```python
from build123d import *

# Parameters (mm, degrees)
F0_R     = 609.6
F0_R_2   = 4.826
F0_R_3   = 3.175
F0_R_4   = 44.9961
F1_DEPTH = 6.35


with BuildPart() as f1:
    # F0 (on Top) → F1 (new body)
    with BuildSketch(Plane.XY):
        Circle(F0_R)
        with Locations((-383.730187, -440.500605)):
            Circle(F0_R_2, mode=Mode.SUBTRACT)
        with Locations((-441.988335, -382.015644)):
            Circle(F0_R_2, mode=Mode.SUBTRACT)
        with Locations((-42.407097, -582.658801)):
            Circle(F0_R_2, mode=Mode.SUBTRACT)
        with Locations((-582.819183, -40.142748)):
            Circle(F0_R_2, mode=Mode.SUBTRACT)
        with Locations((-1.195725, -177.795979)):
            Circle(F0_R_2, mode=Mode.SUBTRACT)
        with Locations((-126.566248, -124.875237)):
            Circle(F0_R_2, mode=Mode.SUBTRACT)
        with Locations((-76.57454, -133.362918)):
            Circle(F0_R_2, mode=Mode.SUBTRACT)
        with Locations((-136.75852, -76.588043)):
            Circle(F0_R_2, mode=Mode.SUBTRACT)
        with Locations((-42.546952, -150.858801)):
            Circle(F0_R_2, mode=Mode.SUBTRACT)
        with Locations((-148.4482, -40.155448)):
            Circle(F0_R_2, mode=Mode.SUBTRACT)
        with Locations((-47.623603, -27.4955)):
            Circle(F0_R_3, mode=Mode.SUBTRACT)
        with Locations((40.142748, -582.819183)):
            Circle(F0_R_2, mode=Mode.SUBTRACT)
        with Locations((382.015644, -441.988335)):
            Circle(F0_R_2, mode=Mode.SUBTRACT)
        with Locations((440.500605, -383.730187)):
            Circle(F0_R_2, mode=Mode.SUBTRACT)
        with Locations((40.155448, -148.4482)):
            Circle(F0_R_2, mode=Mode.SUBTRACT)
        with Locations((76.588043, -136.75852)):
            Circle(F0_R_2, mode=Mode.SUBTRACT)
        with Locations((124.875237, -126.566248)):
            Circle(F0_R_2, mode=Mode.SUBTRACT)
        with Locations((133.362918, -76.57454)):
            Circle(F0_R_2, mode=Mode.SUBTRACT)
        with Locations((0, -54.991)):
            Circle(F0_R_3, mode=Mode.SUBTRACT)
        with Locations((47.623603, -27.4955)):
            Circle(F0_R_3, mode=Mode.SUBTRACT)
        with Locations((150.858801, -42.546952)):
            Circle(F0_R_2, mode=Mode.SUBTRACT)
        with Locations((177.795979, -1.195725)):
            Circle(F0_R_2, mode=Mode.SUBTRACT)
        with Locations((582.658801, -42.407097)):
            Circle(F0_R_2, mode=Mode.SUBTRACT)
        with Locations((-582.658801, 42.407097)):
            Circle(F0_R_2, mode=Mode.SUBTRACT)
        with Locations((-177.795979, 1.195725)):
            Circle(F0_R_2, mode=Mode.SUBTRACT)
        with Locations((-150.858801, 42.546952)):
            Circle(F0_R_2, mode=Mode.SUBTRACT)
        with Locations((-47.623603, 27.4955)):
            Circle(F0_R_3, mode=Mode.SUBTRACT)
        with Locations((-133.362918, 76.57454)):
            Circle(F0_R_2, mode=Mode.SUBTRACT)
        with Locations((-124.875237, 126.566248)):
            Circle(F0_R_2, mode=Mode.SUBTRACT)
        with Locations((-76.588043, 136.75852)):
            Circle(F0_R_2, mode=Mode.SUBTRACT)
        with Locations((-40.155448, 148.4482)):
            Circle(F0_R_2, mode=Mode.SUBTRACT)
        with Locations((-440.500605, 383.730187)):
            Circle(F0_R_2, mode=Mode.SUBTRACT)
        with Locations((-382.015644, 441.988335)):
            Circle(F0_R_2, mode=Mode.SUBTRACT)
        with Locations((-40.142748, 582.819183)):
            Circle(F0_R_2, mode=Mode.SUBTRACT)
        Circle(F0_R_4, mode=Mode.SUBTRACT)
        with Locations((47.623603, 27.4955)):
            Circle(F0_R_3, mode=Mode.SUBTRACT)
        with Locations((0, 54.991)):
            Circle(F0_R_3, mode=Mode.SUBTRACT)
        with Locations((148.4482, 40.155448)):
            Circle(F0_R_2, mode=Mode.SUBTRACT)
        with Locations((42.546952, 150.858801)):
            Circle(F0_R_2, mode=Mode.SUBTRACT)
        with Locations((136.75852, 76.588043)):
            Circle(F0_R_2, mode=Mode.SUBTRACT)
        with Locations((76.57454, 133.362918)):
            Circle(F0_R_2, mode=Mode.SUBTRACT)
        with Locations((126.566248, 124.875237)):
            Circle(F0_R_2, mode=Mode.SUBTRACT)
        with Locations((1.195725, 177.795979)):
            Circle(F0_R_2, mode=Mode.SUBTRACT)
        with Locations((582.819183, 40.142748)):
            Circle(F0_R_2, mode=Mode.SUBTRACT)
        with Locations((42.407097, 582.658801)):
            Circle(F0_R_2, mode=Mode.SUBTRACT)
        with Locations((441.988335, 382.015644)):
            Circle(F0_R_2, mode=Mode.SUBTRACT)
        with Locations((383.730187, 440.500605)):
            Circle(F0_R_2, mode=Mode.SUBTRACT)
    extrude(amount=F1_DEPTH)


solid = f1.part
```
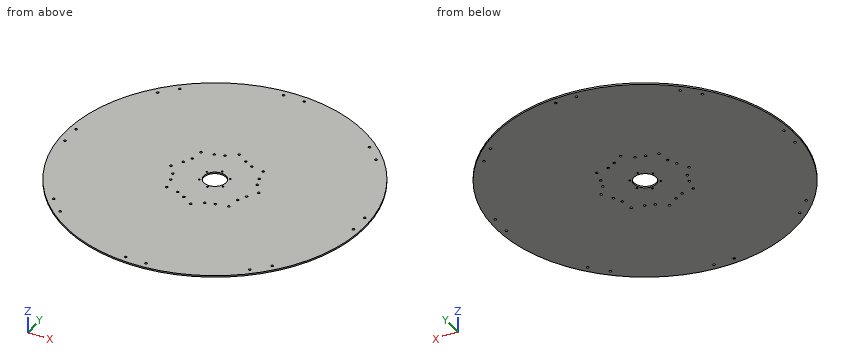
Work out the finished part from the listing and answer in its coordinate system (mm). Round coordinates to 2 decimals unless told otherwise and drop trailing zeros. Loops run counter-clockwise (first coordinate to the right, second up) from the corner with the lowest first, then second, coordinate; pieces in that order, holes last. Notation, with made-up numbers: M -12.75,61 L 34.25,61 A11 ccw 34.25,82 Z; hole C -28,-24.75 d7. An arc over 180 degrees is marked long. One line per question, with ' | ' between items.
Q1. Find section B-B, the plane y = 226. Give the vertices of the cut face in (x, z).
Conclusion:
outline: M -566.16,0 L 566.16,0 L 566.16,6.35 L -566.16,6.35 Z
Q2. Find section C-C, the plane z = 4. State how many separate pieces and enclosed holes the cut face has, then the cut area to 3 significant figures.
Conclusion:
separate pieces: 1 | enclosed holes: 47 | area: 1,160,000 mm2
Q3. Find section A-A, the plane x = -523.5. Give the vertices of the cut face in (y, z), then the cut area to 3 significant figures.
Conclusion:
outline: M -312.35,0 L 312.35,0 L 312.35,6.35 L -312.35,6.35 Z | area: 3,970 mm2
Q4. Consider line 1 along X through (y, z) = (-382, 2); line 2 along X through (y, z) = (-386, 3); line 3 along X through (y, z) = (-174, 0.5). Determine where each line is inside the solid, lowest interval first. Write a range as from..to.
Conclusion:
line 1: x = -475.07..-446.81, -437.16..436, 445.01..475.07 | line 2: x = -471.82..-444.71, -439.27..436.24, 444.76..471.82 | line 3: x = -584.24..-4.18, 1.78..584.24
Q5. Each of these flat-tipped pins is pushed along its axis until it touches: pin 1 Ø2 at (y, z) = (-146, 3) entering from +X; pin 2 Ø1 at (y, z) = (-371, 3.5) entering from -X; pin 3 Ø1.5 at (y, z) = (407.5, 1) entering from -X; pin 4 Ø6 at (x, y) = (582.82, 40.14) entering from +Z. Where does it stop, or does it pass through?
Conclusion:
pin 1: stops at x = 592.1 | pin 2: stops at x = -484.09 | pin 3: stops at x = -454.06 | pin 4: passes through
